Read the model definition and answer for the solid it produces. Units are mm, in the model's axes. Face numbers are marked on the shaded views. A direction names the side the tool comes from. Give positions to 0.01 mm unless a question says otherwise; leave off trailing zeros. Order: outer loops, then holes, each group sorted by start corner. A loop starts at its lowest first (then second) coordinate and runs counter-clockwise, first axis right, second up. Notation, with made-up numbers: (15.5, -22.5) - (43.5, -22.5) arc R24 ccw to (43.5, 10.5) - close; hole circle Ø6 at (11.5, 5.25). An arc over 180 degrees is marked (long way). Return JSON: item names as keys, results as strings.
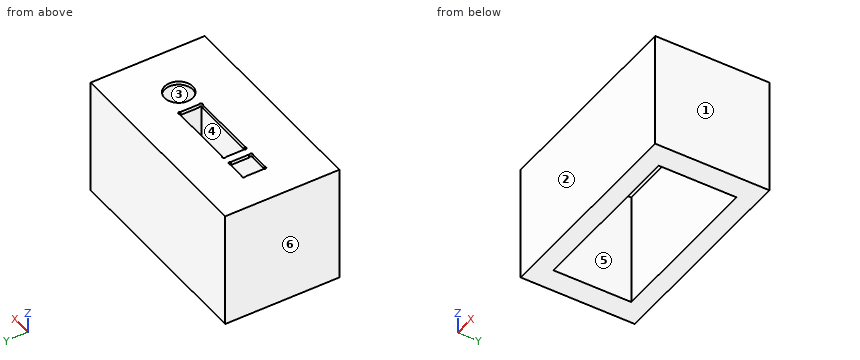
```python
from build123d import *

# Parameters (mm, degrees)
F0_W     = 92
F0_H     = 50
F0_W_2   = 72
F0_H_2   = 34.1
F1_DEPTH = 50
F0_R     = 6.2
F2_DEPTH = 1.5


with BuildPart() as f1:
    # F0 (on Top) → F1 (new body)
    with BuildSketch(Plane.XY):
        Rectangle(F0_W, F0_H)
        Rectangle(F0_W_2, F0_H_2, mode=Mode.SUBTRACT)
    extrude(amount=-F1_DEPTH)

    # F0 (on Top) → F2 (join)
    with BuildSketch(Plane.XY):
        Rectangle(F0_W, F0_H)
        Rectangle(F0_W_2, F0_H_2, mode=Mode.SUBTRACT)
        Rectangle(F0_W_2, F0_H_2)
        with BuildLine():
            ThreePointArc((-30.6, 6.18934), (-30.81967, 6.71967), (-30.6, 7.25))
            ThreePointArc((-30.6, 7.25), (-30.06967, 7.46967), (-29.53934, 7.25))
            Line((-29.53934, 7.25), (-21.66066, 7.25))
            ThreePointArc((-21.66066, 7.25), (-21.13033, 7.46967), (-20.6, 7.25))
            ThreePointArc((-20.6, 7.25), (-20.43742, 7.006682), (-20.38033, 6.71967))
            ThreePointArc((-20.38033, 6.71967), (-20.43742, 6.432657), (-20.6, 6.18934))
            Line((-20.6, 6.18934), (-20.6, -1.78934))
            ThreePointArc((-20.6, -1.78934), (-20.43742, -2.032657), (-20.38033, -2.31967))
            ThreePointArc((-20.38033, -2.31967), (-20.43742, -2.606682), (-20.6, -2.85))
            ThreePointArc((-20.6, -2.85), (-21.13033, -3.06967), (-21.66066, -2.85))
            Line((-21.66066, -2.85), (-29.53934, -2.85))
            ThreePointArc((-29.53934, -2.85), (-30.06967, -3.06967), (-30.6, -2.85))
            ThreePointArc((-30.6, -2.85), (-30.81967, -2.31967), (-30.6, -1.78934))
            Line((-30.6, -1.78934), (-30.6, 6.18934))
        make_face(mode=Mode.SUBTRACT)
        with BuildLine():
            ThreePointArc((-17.2, 6.18934), (-17.41967, 6.71967), (-17.2, 7.25))
            ThreePointArc((-17.2, 7.25), (-16.66967, 7.46967), (-16.13934, 7.25))
            Line((-16.13934, 7.25), (12.73934, 7.25))
            ThreePointArc((12.73934, 7.25), (13.26967, 7.46967), (13.8, 7.25))
            ThreePointArc((13.8, 7.25), (13.96258, 7.006682), (14.01967, 6.71967))
            ThreePointArc((14.01967, 6.71967), (13.96258, 6.432657), (13.8, 6.18934))
            Line((13.8, 6.18934), (13.8, -1.78934))
            ThreePointArc((13.8, -1.78934), (13.96258, -2.032657), (14.01967, -2.31967))
            ThreePointArc((14.01967, -2.31967), (13.96258, -2.606682), (13.8, -2.85))
            ThreePointArc((13.8, -2.85), (13.26967, -3.06967), (12.73934, -2.85))
            Line((12.73934, -2.85), (-16.13934, -2.85))
            ThreePointArc((-16.13934, -2.85), (-16.66967, -3.06967), (-17.2, -2.85))
            ThreePointArc((-17.2, -2.85), (-17.41967, -2.31967), (-17.2, -1.78934))
            Line((-17.2, -1.78934), (-17.2, 6.18934))
        make_face(mode=Mode.SUBTRACT)
        with Locations((23.8, 0.65)):
            Circle(F0_R, mode=Mode.SUBTRACT)
    extrude(amount=F2_DEPTH)


solid = f1.part
```
Q1. Determine the mould class of the marked faces 1, 2, 3 and 4 for opening direction Y: released by +Y, released by -Y, zero draft, split by the parting line, or undercut.
Values:
{"face 1": "zero draft", "face 2": "released by -Y", "face 3": "undercut", "face 4": "undercut"}
Q2. A cutting plane is placed at B-B (y = 0.65). Write down the section's boundary in (x, z), and give its area (3 significant figures).
Values:
{"outline": "(-46, -50) - (-36, -50) - (-36, 0) - (-30.6, 0) - (-30.6, 1.5) - (-46, 1.5) - close; (-20.6, 0) - (-17.2, 0) - (-17.2, 1.5) - (-20.6, 1.5) - close; (13.8, 0) - (17.6, 0) - (17.6, 1.5) - (13.8, 1.5) - close; (30, 0) - (36, 0) - (36, -50) - (46, -50) - (46, 1.5) - (30, 1.5) - close", "area": "1,060 mm²"}
Q3. Given pin 1 (8 mm diameter, centred on x = -31.5, y = 2, fed in from -Z), flat-ended and moving along its own axis, determine where the tip first touches the part or whether it passes through.
Values:
{"pin 1": "stops at z = 0"}
Q4. Consider L1, parallel to X at y = 7, z = -7; L2, parallel to Y at x = -6, z = -42; L3, parallel to Y at x = 23.8, z = 0.45. Determine where each line is inside the solid, lowest interval first.
Values:
{"L1": "x = -46 to -36, 36 to 46", "L2": "y = -25 to -17.05, 17.05 to 25", "L3": "y = -25 to -5.55, 6.85 to 25"}
Q5. A cutting plane is placed at A-A (x = 23.8). Write down the section's boundary in (y, z), and give its area (3 significant figures).
Values:
{"outline": "(-25, -50) - (-17.05, -50) - (-17.05, 0) - (-5.55, 0) - (-5.55, 1.5) - (-25, 1.5) - close; (6.85, 0) - (17.05, 0) - (17.05, -50) - (25, -50) - (25, 1.5) - (6.85, 1.5) - close", "area": "851 mm²"}
Q6. For the marked faces 5 and 6, determine the directions among +Z, -Z, +X, -X, +Y, -Y from which every point of the face is accessible in a straight line to the end or side of a thin tool.
Values:
{"face 5": "-Z", "face 6": "+Z, -Z, -X, +Y, -Y"}
Q7. A cutting plane is placed at D-D (y = -7). Write down the section's boundary in (x, z), and give its area (3 significant figures).
Values:
{"outline": "(-46, -50) - (-36, -50) - (-36, 0) - (36, 0) - (36, -50) - (46, -50) - (46, 1.5) - (-46, 1.5) - close", "area": "1,140 mm²"}
Q8. A cutting plane is placed at C-C (z = -21.5). Write down the section's boundary in (x, y), and give its area (3 significant figures).
Values:
{"outline": "(-46, -25) - (46, -25) - (46, 25) - (-46, 25) - close; hole (-36, -17.05) - (36, -17.05) - (36, 17.05) - (-36, 17.05) - close", "area": "2,140 mm²"}
